Print and shaded views of the part. All mm, measured from the part's lowest x, y and z. Coordinates: 2 decimals unless noted, no trailing zeros. Order: outer loops, then holes, each group sorted by start corner. A loop starts at its lowest first (then second) coordinate and runs counter-clockwise, first axis right, second up. Notation, with made-up numbers: M 2,16.5 L 8,16.5 A28 cw 8,36.5 Z; hole C 9.5,-17 d3. An arc over 180 degrees is marked long. Return JSON: item names as keys, results as strings.
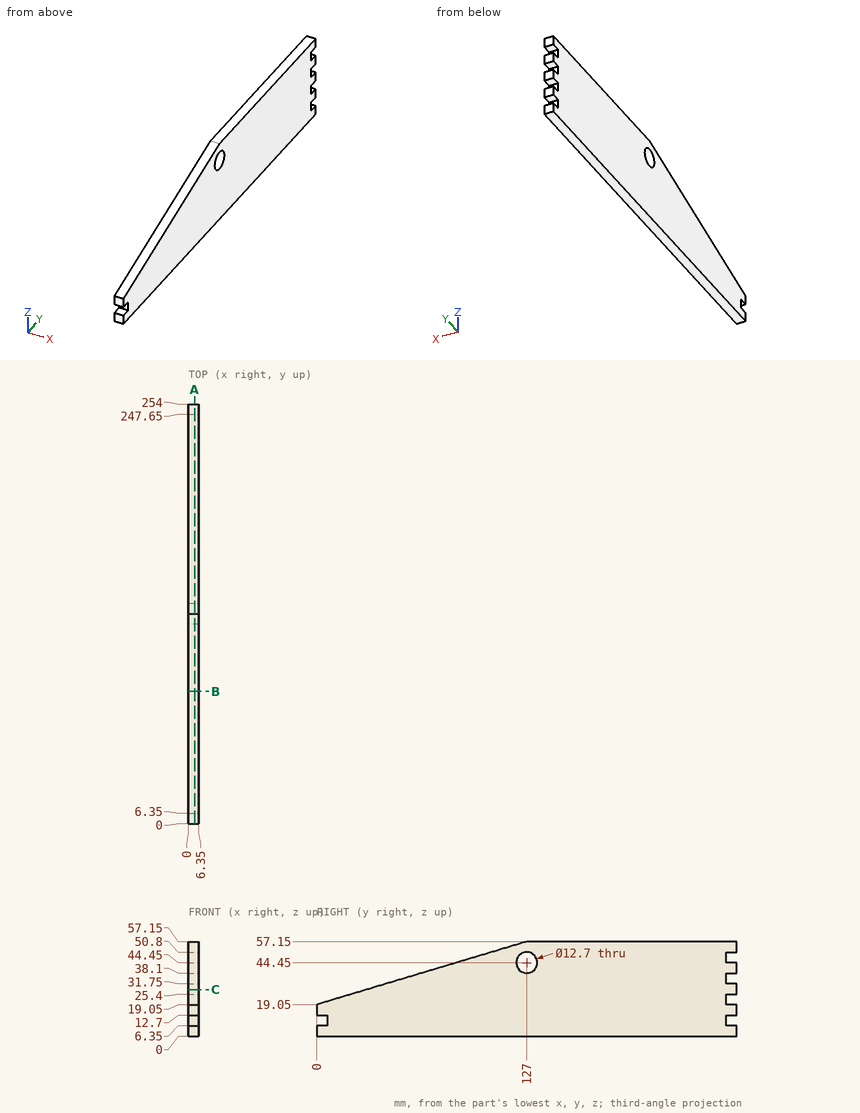
Item 1: Drop flat-ended pins along their axis: pin 1 Ø3 at (x, z) = (2.5, 23) entering from +Y; pin 2 Ø1.9 at (x, y) = (4, 3) entering from +Z (3 decimals). Give the stop position or say it passes through.
Check result:
{"pin 1": "stops at y = 247.65", "pin 2": "stops at z = 20.235"}
Item 2: Wall check: line 1 (Y direction, x = 1.25, z = 10); line 2 (Z direction, x = 3.5, y = 68); line 3 (Z direction, x = 1.75, y = 22.5). Give the ranges that are in metal, low to high.
Check result:
{"line 1": "y = 6.35 to 247.65", "line 2": "z = 0 to 39.45", "line 3": "z = 0 to 25.8"}
Item 3: Saw through at A-A (x = 3.75). Write the cut outline in (y, z), and give its area (3 significant figures).
Check result:
{"outline": "M 0,0 L 254,0 L 254,6.35 L 247.65,6.35 L 247.65,12.7 L 254,12.7 L 254,19.05 L 247.65,19.05 L 247.65,25.4 L 254,25.4 L 254,31.75 L 247.65,31.75 L 247.65,38.1 L 254,38.1 L 254,44.45 L 247.65,44.45 L 247.65,50.8 L 254,50.8 L 254,57.15 L 127,57.15 L 0,19.05 L 0,12.7 L 6.35,12.7 L 6.35,6.35 L 0,6.35 Z; hole C 127,44.45 d12.7", "area": "11,800 mm2"}
Item 4: Saw through at C-C (z = 28). Write the cut outline in (x, y).
Check result:
{"outline": "M 0,29.83 L 6.35,29.83 L 6.35,254 L 0,254 Z"}
Item 5: Saw through at B-B (y = 80). Write the cut outline in (x, z).
Check result:
{"outline": "M 0,0 L 6.35,0 L 6.35,43.05 L 0,43.05 Z"}
